```python
from build123d import *

# Parameters (mm, degrees)
F0_W      = 165.363372
F0_H      = 127
F1_DEPTH  = 9.525
F2_W      = 50.8
F2_H      = 50.800003
F3_DEPTH  = 63.5
F4_W      = 50.8
F4_H      = 50.8
F5_DEPTH  = 63.5
F6_R      = 25.4
F7_R      = 19.05
F8_DEPTH  = 63.501
F9_R      = 19.05
F10_DEPTH = 63.501
F11_R     = 19.05
F12_DEPTH = 9.526
F13_R     = 6.35
F14_DEPTH = 44.45


with BuildPart() as f1:
    # F0 (on Front) → F1 (new body)
    with BuildSketch(Plane.XZ):
        Rectangle(F0_W, F0_H)
    extrude(amount=F1_DEPTH)

    # F2 (on Front) → F3 (join)
    with BuildSketch(Plane.XZ):
        with Locations((56.94912, 37.684852)):
            Rectangle(F2_W, F2_H)
    extrude(amount=-F3_DEPTH)

    # F4 (on face) → F5 (join)
    with BuildSketch(Plane(origin=(0, 0, 0), x_dir=(-1, 0, 0), z_dir=(0, 1, 0))):
        with Locations((57.281686, 38.1)):
            Rectangle(F4_W, F4_H)
    extrude(amount=F5_DEPTH)

    # F6
    f6_edges = [f1.edges().sort_by_distance(p)[0] for p in [
        (31.54912, 31.75, 12.284851),
        (-31.881686, 31.75, 12.7),
    ]]
    fillet(f6_edges, radius=F6_R)

    # F7 (on Front) → F8 (cut, through all)
    with BuildSketch(Plane.XZ):
        Circle(F7_R)
    extrude(amount=-F8_DEPTH, mode=Mode.SUBTRACT)

    # F9 (on Front) → F10 (cut, through all)
    with BuildSketch(Plane.XZ):
        Circle(F9_R)
    extrude(amount=-F10_DEPTH, mode=Mode.SUBTRACT)

    # F11 (on Front) → F12 (cut, through all)
    with BuildSketch(Plane.XZ):
        Circle(F11_R)
    extrude(amount=F12_DEPTH, mode=Mode.SUBTRACT)

    # F13 (on face) → F14 (cut)
    with BuildSketch(Plane(origin=(0, 63.5, 0), x_dir=(-1, 0, 0), z_dir=(0, 1, 0))):
        with Locations((-56.94912, 37.684854)):
            Circle(F13_R)
        with Locations((57.281686, 38.1)):
            Circle(F13_R)
    extrude(amount=-F14_DEPTH, mode=Mode.SUBTRACT)


solid = f1.part
```
Could you check a few things on this model? Use its own coordinates, in mm. A direction names the side the tool comes from. Give positions to 0.01 mm unless a question says otherwise; leave off trailing zeros. Order: outer loops, then holes, each group sorted by start corner. A loop starts at its lowest first (then second) coordinate and runs counter-clockwise, first axis right, second up.
Q1. Suppose I cut it at D-D, the plane y = 3.5. Write out the boundary of the cut face in (x, z), and give its area (3 significant figures).
Q2. For faces 1 (the flat face through (57, 19.05, 38)), 2 (the flat face through (31.549, 31, 50)), 3 (the cylindrical face through (-39.125, 32.194, 20.338)), 4 (the flat face through (57, 31, 63.085)), 5 (the flat face through (-70, 31, 12.7)), which set-ups out of +Z, -Z, +X, -X, +Y, -Y let a thin tool reach every point of the face, with its end or its side?
Q3. Suppose I cut it at A-A, the plane y = 27. Write out the boundary of the cut face in (x, z), and give its area (3 significant figures).
Q4. Suppose I cut it at C-C, the plane z = 0. Write out the boundary of the cut face in (x, y) (3 decimals).
Q5. I'm going to push flat-ended pins straight in: P1, Ø20.5, axis at x = 67, y = 40, coming from the -Z side; P2, Ø6.5, axis at x = 58, z = 40, coming from the +Y side; P3, Ø5, axis at x = -41, z = -12.5, coming from the +Y side. Where does each tip first touch, or does it pass through?
Q6. We'd pull the mould along X, two halves only. Please class faces 6 (the flat face through (-82.682, 26, 27)), 7 (the flat face through (62, 63.5, 44)), 8 (the flat face through (-1, 0, -27)): +X half, -X half, draft (parallel to the pull), parting line (faces both ways), or undercut.
Q7. If I drill on line 1 along X through (y, z) = (-2, 0); line 2 along X through (y, z) = (42, 38); line 3 along X through (y, z) = (54.5, 37), over which ranges is the centre line in solid material (lowest first)?
Q8. Suppose I cut it at B-B, the plane x = 0. Write out the boundary of the cut face in (y, z) (3 decimals), and give its area (3 significant figures).
Solution:
1. outline: (-82.68, 12.7) - (-57.28, 12.7) arc R25.4 ccw to (-31.88, 38.1) - (-31.88, 63.5) - (-82.68, 63.5) - close; (31.55, 37.68) arc R25.4 ccw to (56.95, 12.28) - (82.35, 12.28) - (82.35, 63.08) - (31.55, 63.08) - close
1. area: 4,880 mm2
2. face 1: +Y
2. face 2: +Z, -Z, +Y
2. face 3: -Z, +Y
2. face 4: +Z, +X, +Y
2. face 5: -Z, -X, +Y
3. outline: (-82.68, 12.7) - (-57.28, 12.7) arc R25.4 ccw to (-31.88, 38.1) - (-31.88, 63.5) - (-82.68, 63.5) - close; (31.55, 37.68) arc R25.4 ccw to (56.95, 12.28) - (82.35, 12.28) - (82.35, 63.08) - (31.55, 63.08) - close; hole circle Ø12.7 at (-57.28, 38.1); hole circle Ø12.7 at (56.95, 37.68)
3. area: 4,630 mm2
4. outline: (-82.682, -9.525) - (-19.05, -9.525) - (-19.05, 0) - (-82.682, 0) - close; (19.05, -9.525) - (82.682, -9.525) - (82.682, 0) - (19.05, 0) - close
5. P1: stops at z = 12.28
5. P2: stops at y = 19.05
5. P3: stops at y = 0
6. face 6: -X half
6. face 7: draft
6. face 8: undercut
7. line 1: x = -82.68 to -19.05, 19.05 to 82.68
7. line 2: x = -82.68 to -63.63, -50.93 to -31.88, 31.55 to 50.61, 63.29 to 82.35
7. line 3: x = -82.68 to -63.54, -51.03 to -31.91, 31.56 to 50.64, 63.26 to 82.35
8. outline: (-9.525, -63.5) - (0, -63.5) - (0, -19.05) - (-9.525, -19.05) - close; (-9.525, 19.05) - (0, 19.05) - (0, 63.5) - (-9.525, 63.5) - close
8. area: 847 mm2
